from build123d import *

# Parameters (mm, degrees)
BOSS_EXTRUDE1_DEPTH = 4.7371
CUT_EXTRUDE1_REACH  = 25.851
SKETCH4_R           = 2.38125
SKETCH5_R           = 2.38125
CUT_EXTRUDE2_DEPTH  = 10.525


with BuildPart() as part:
    # Sketch3 → Boss-Extrude1 (new body, symmetric)
    with BuildSketch(Plane.XY):
        Polygon((2.3876, -9.68375), (-2.3876, -9.68375), (-2.3876, 4.83235), (-4.7625, 4.83235), (-4.7625, -19.01825), (4.7625, -19.01825), (4.7625, 4.83235), (2.3876, 4.83235), align=None)
    extrude(amount=BOSS_EXTRUDE1_DEPTH, both=True)

    # Sketch4 → Cut-Extrude1 (cut, up to next)
    with BuildSketch(Plane.XZ.offset(19.01825), mode=Mode.PRIVATE) as cut_extrude1_sk1:
        Circle(SKETCH4_R)
    cut_extrude1_tool1 = extrude(cut_extrude1_sk1.sketch, amount=-CUT_EXTRUDE1_REACH, mode=Mode.PRIVATE) & part.part
    add(cut_extrude1_tool1.solids().sort_by_distance((0, -19.01825, 0))[0], mode=Mode.SUBTRACT)

    # Sketch5 → Cut-Extrude2 (cut, through all)
    with BuildSketch(Plane(origin=(4.7625, 0, 0), x_dir=(0, 0, -1), z_dir=(1, 0, 0))):
        Circle(SKETCH5_R)
    extrude(amount=-CUT_EXTRUDE2_DEPTH, mode=Mode.SUBTRACT)


solid = part.part
Source: CAD feature listing. Evaluate the final solid. Frame: model axes, mm. A direction names the side the tool comes from. Coordinates: 2 decimals unless noted, no trailing zeros. Loops run counter-clockwise (first coordinate to the right, second up) from the corner with the lowest first, then second, coordinate; pieces in that order, holes last. Notation, with made-up numbers: M 57.25,-39.75 L 84.25,-39.75 A22 ccw 84.25,-28.75 Z; hole C 49.5,45 d9. An arc over 180 degrees is marked long. Answer in a Markdown table with one row per item.
Q1. First-contact query: pin 1 (2.5 mm diameter, centred on x = 1, z = 2, fed in from +Y); pin 2 (4.5 mm diameter, centred on x = 0, z = 0, fed in from +Y). Flat tips, straight axial feed; report the tip coordinate or a pass-through.
Answers below:
| item | result |
|---|---|
| pin 1 | stops at y = -9.68 |
| pin 2 | passes through |
Q2. Section C-C on x = 0. Return the cut outline in (y, z).
Answers below:
| item | result |
|---|---|
| outline | M -19.02,-4.74 L -9.68,-4.74 L -9.68,-2.38 L -19.02,-2.38 Z; M -19.02,2.38 L -9.68,2.38 L -9.68,4.74 L -19.02,4.74 Z |
Q3. Set-up query: faces 1 (the flat face through (4, 4.832, 0)), 2 (the flat face through (2, -9.684, 2)). Return all of +Z, -Z, +X, -X, +Y, -Y with unobstructed straight access to the full face (end or side cutting, diameter ignored); none if empty.
Answers below:
| item | result |
|---|---|
| face 1 | +Z, -Z, +X, -X, +Y |
| face 2 | +Z, -Z, +Y |
Q4. Draft query along Z for faces 3 (the flat face through (2.388, -2.3, 1.1)), 4 (the cylindrical face through (3.59, -1.45, 1.89)), 5 (the flat face through (0, -12, -4.737)). Return one class per face: pulls with the +Z half, pulls with the -Z half, needs draft (parallel to the pull), parting line crosses it, or undercut.
Answers below:
| item | result |
|---|---|
| face 3 | needs draft |
| face 4 | undercut |
| face 5 | pulls with the -Z half |
Q5. Section D-D on y = -5.75. Return the cut outline in (x, z).
Answers below:
| item | result |
|---|---|
| outline | M -4.76,-4.74 L -2.39,-4.74 L -2.39,4.74 L -4.76,4.74 Z; M 2.39,-4.74 L 4.76,-4.74 L 4.76,4.74 L 2.39,4.74 Z |
Q6. Section B-B on z = 0. State how many separate pieces and enclosed holes the cut face has, plus the area to 3 significant figures.
Answers below:
| item | result |
|---|---|
| separate pieces | 4 |
| enclosed holes | 0 |
| area | 90.8 mm^2 |
Q7. Section A-A on y = 0. Return the cut outline in (x, z), plus the area to 3 significant figures.
Answers below:
| item | result |
|---|---|
| outline | M -4.76,-4.74 L -2.39,-4.74 L -2.39,-2.38 L -4.76,-2.38 Z; M -4.76,2.38 L -2.39,2.38 L -2.39,4.74 L -4.76,4.74 Z; M 2.39,-4.74 L 4.76,-4.74 L 4.76,-2.38 L 2.39,-2.38 Z; M 2.39,2.38 L 4.76,2.38 L 4.76,4.74 L 2.39,4.74 Z |
| area | 22.4 mm^2 |
Q8. Ray query, probe 1 along Z at (x, y) = (0, -15); probe 2 along X at (y, z) = (-4.5, 1.25); probe 3 along Y at (x, z) = (4.2, 0). Return the intervals inside material, ascending. Write a range as from..to.
Answers below:
| item | result |
|---|---|
| probe 1 | z = -4.74..-2.38, 2.38..4.74 |
| probe 2 | x = -4.76..-2.39, 2.39..4.76 |
| probe 3 | y = -19.02..-2.38, 2.38..4.83 |
